CAD build for the part. Positions are in the model's coordinates, mm. A direction names the side the tool comes from. Round coordinates to 2 decimals unless told otherwise and drop trailing zeros. Write each loop counter-clockwise with the first axis right and the second up, starting at its lowest first coordinate (ties: lowest second). Pieces come first, ordered by that corner, then holes. Notation, with made-up numbers: (-37.75, 88) - (-26.75, 88) arc R6 cw to (-26.75, 92) - close; hole circle Ø3 at (43.25, 36). An arc over 180 degrees is marked (long way). Answer in a Markdown table with one row per item.
```python
from build123d import *

# Parameters (mm, degrees)
ESQUISSE1_W                  = 58.7375
ESQUISSE1_H                  = 15.24
BOSS_EXTRU_1_DEPTH           = 3.175
ESQUISSE1_3_W                = 4.7625
ESQUISSE1_3_H                = 15.24
BOSS_EXTRU_2_DEPTH           = 25.4
ENL_V_MAT_EXTRU_1_DEPTH      = 69.814783295
ENL_V_MAT_EXTRU_1_DEPTH_BACK = 69.814783295
CONG_1_R                     = 6.35
CONG_2_R                     = 1.27


with BuildPart() as part:
    # Esquisse1 → Boss.-Extru.1 (new body)
    with BuildSketch(Plane(origin=(0, 0, 0), x_dir=(1, 0, 0), z_dir=(0, 1, 0))):
        with Locations((2.38125, 0)):
            Rectangle(ESQUISSE1_W, ESQUISSE1_H)
        with BuildLine():
            ThreePointArc((19.05, 2.2479), (21.2979, 0), (19.05, -2.2479))
            Line((19.05, -2.2479), (-14.2875, -2.2479))
            ThreePointArc((-14.2875, -2.2479), (-16.5354, 0), (-14.2875, 2.2479))
            Line((-14.2875, 2.2479), (19.05, 2.2479))
        make_face(mode=Mode.SUBTRACT)
    extrude(amount=BOSS_EXTRU_1_DEPTH)

    # Esquisse1<3> → Boss.-Extru.2 (add)
    with BuildSketch(Plane(origin=(0, 0, 0), x_dir=(1, 0, 0), z_dir=(0, 1, 0))):
        with Locations((-29.36875, 0)):
            Rectangle(ESQUISSE1_3_W, ESQUISSE1_3_H)
    extrude(amount=BOSS_EXTRU_2_DEPTH)

    # Esquisse3 → Enlèv. mat.-Extru.1 (cut, two sides: drawn at the far end of the back side and taken through both)
    with BuildSketch(Plane.ZY.offset(31.75).offset(-ENL_V_MAT_EXTRU_1_DEPTH_BACK)):
        with BuildLine():
            Line((2.2479, 19.05), (2.2479, 9.525))
            ThreePointArc((2.2479, 9.525), (0, 7.2771), (-2.2479, 9.525))
            Line((-2.2479, 9.525), (-2.2479, 19.05))
            ThreePointArc((-2.2479, 19.05), (0, 21.2979), (2.2479, 19.05))
        make_face()
    extrude(amount=ENL_V_MAT_EXTRU_1_DEPTH + ENL_V_MAT_EXTRU_1_DEPTH_BACK, mode=Mode.SUBTRACT)

    # Congé1
    # the kernel refuses this fillet: 6.35 mm, written as the material it adds along each edge
    with BuildSketch(Plane(origin=(-26.9875, 3.175, -7.62), x_dir=(1, 0, 0), z_dir=(0, 0, 1))) as cong_1_piece_1_section:
        with BuildLine():
            CenterArc((CONG_1_R, CONG_1_R), CONG_1_R, 180, 90)
            Line((0, CONG_1_R), (0, 0))
            Line((0, 0), (CONG_1_R, 0))
        make_face()
    cong_1_piece_1 = extrude(amount=15.24, mode=Mode.PRIVATE)
    cong_1_piece_1 = cong_1_piece_1 - Plane(origin=(-25.549891024, 9.525, 0), x_dir=(0, 0, 1), z_dir=(1, 0, 0)) * Cylinder(2.2479, 56, mode=Mode.PRIVATE)
    add(cong_1_piece_1)
    # the kernel refuses this fillet: 6.35 mm, written as the material it takes off along each edge
    with BuildSketch(Plane(origin=(31.75, -15.875, 7.62), x_dir=(0, 0, -1), z_dir=(0, 1, 0)), Plane(origin=(31.75, -15.875, -7.62), x_dir=(-1, 0, 0), z_dir=(0, 1, 0))) as cong_1_2_piece_1:
        with BuildLine():
            CenterArc((CONG_1_R, CONG_1_R), CONG_1_R, 180, 90)
            Line((0, CONG_1_R), (0, 0))
            Line((0, 0), (CONG_1_R, 0))
        make_face()
    extrude(amount=34.925, mode=Mode.SUBTRACT)
    with BuildSketch(Plane(origin=(-11.1125, 25.4, -7.62), x_dir=(0, -1, 0), z_dir=(-1, 0, 0))) as cong_1_2_piece_2:
        with BuildLine():
            CenterArc((CONG_1_R, CONG_1_R), CONG_1_R, 180, 90)
            Line((0, CONG_1_R), (0, 0))
            Line((0, 0), (CONG_1_R, 0))
        make_face()
    extrude(amount=36.5125, mode=Mode.SUBTRACT)
    with BuildSketch(Plane(origin=(-47.625, 25.4, 7.62), x_dir=(0, 0, -1), z_dir=(1, 0, 0))) as cong_1_2_piece_3:
        with BuildLine():
            CenterArc((CONG_1_R, -CONG_1_R), CONG_1_R, 90, 90)
            Line((0, -CONG_1_R), (0, 0))
            Line((0, 0), (CONG_1_R, 0))
        make_face()
    extrude(amount=36.5125, mode=Mode.SUBTRACT)

    # Congé2
    cong_2_edges = [part.edges().sort_by_distance(p)[0] for p in [
        (-3.175, 0, -7.62),
        (-3.175, 0, 7.62),
        (-31.75, 0, 0),
        (2.38125, 3.175, 7.62),
        (31.75, 3.175, 0),
        (2.38125, 3.175, -7.62),
        (29.890128061, 3.175, -5.760128061),
        (29.890128061, 3.175, 5.760128061),
        (-26.9875, 14.2875, -7.62),
        (-26.9875, 25.4, 0),
        (-26.9875, 14.2875, 7.62),
        (-26.9875, 23.540128061, 5.760128061),
        (-26.9875, 23.540128061, -5.760128061),
        (31.75, 0, 0),
        (29.890128061, 0, -5.760128061),
        (29.890128061, 0, 5.760128061),
        (-31.75, 9.525, 7.62),
        (-31.75, 9.525, -7.62),
        (-31.75, 25.4, 0),
        (-31.75, 23.540128061, 5.760128061),
        (-31.75, 23.540128061, -5.760128061),
        (-25.127628061, 5.034871939, 7.62),
        (-25.127628061, 5.034871939, -7.62),
    ]]
    fillet(cong_2_edges, radius=CONG_2_R)


solid = part.part
```
Q1. Saw through at C-C on z = 0. Count the separate pieces of the cut face and the enclosed holes in it, then the cut area to 3 significant figures.
Computed:
| item | result |
|---|---|
| separate pieces | 3 |
| enclosed holes | 0 |
| area | 127 mm2 |
Q2. Drill centre lines: line 1 (X direction, y = 22.5, z = 1); line 2 (Z direction, x = 20.5, y = 3); line 3 (Y direction, x = 0, z = 4) (3 decimals). Where is each one in solid material? Low to high.
Computed:
| item | result |
|---|---|
| line 1 | x = -31.75 to -26.99 |
| line 2 | z = -6.99 to -1.72, 1.72 to 6.99 |
| line 3 | y = 0 to 3.175 |
Q3. Saw through at B-B on x = 3. List the corners of the cut face in (y, z) (3 decimals).
Computed:
| item | result |
|---|---|
| outline | (0, -6.35) arc R1.27 ccw to (1.27, -7.62) - (1.905, -7.62) arc R1.27 ccw to (3.175, -6.35) - (3.175, -2.248) - (0, -2.248) - close; (0, 2.248) - (3.175, 2.248) - (3.175, 6.35) arc R1.27 ccw to (1.905, 7.62) - (1.27, 7.62) arc R1.27 ccw to (0, 6.35) - close |
Q4. Pull direction Y, two halves, no side cores. Call faces 1 (the cylindrical face through (-29.4, 23.6, 5.7)), 2 (the flat face through (-26.987, 17, -3)), 3 (the cylindrical face through (-29.335, 21.297, -0.049)), 4 (the cylindrical face through (-29.127, 7.278, 0.049)): released by +Y, released by -Y, zero draft, split by the parting line, or undercut.
Computed:
| item | result |
|---|---|
| face 1 | released by +Y |
| face 2 | zero draft |
| face 3 | undercut |
| face 4 | undercut |
Q5. Flat gauge pins, fed straight in: pin 1 (4 mm diameter, centred on y = 17, z = 1, fed in from +X); pin 2 (6.5 mm diameter, centred on x = 14.5, z = -0.5, fed in from +Y) (3 decimals). Where does each tip first touch, or does it go through?
Computed:
| item | result |
|---|---|
| pin 1 | stops at x = -26.99 |
| pin 2 | stops at y = 3.175 |
Q6. Saw through at A-A on y = 15. List the corners of the cut face in (x, z).
Computed:
| item | result |
|---|---|
| outline | (-31.75, -6.35) arc R1.27 ccw to (-30.48, -7.62) - (-28.26, -7.62) arc R1.27 ccw to (-26.99, -6.35) - (-26.99, -2.25) - (-31.75, -2.25) - close; (-31.75, 2.25) - (-26.99, 2.25) - (-26.99, 6.35) arc R1.27 ccw to (-28.26, 7.62) - (-30.48, 7.62) arc R1.27 ccw to (-31.75, 6.35) - close |
Q7. 3-axis set-ups, long thin cutter, end or side, ignore diameter. For faces 5 (the flat face through (5, 3.175, -3)), 6 (the cylindrical face through (2.7, 2.81, 7.24)), 7 (the cylindrical face through (-31.368, 10.036, -7.258)): which of +Z, -Z, +X, -X, +Y, -Y reach the whole face in a straight line?
Computed:
| item | result |
|---|---|
| face 5 | +Z, -Z, +X, +Y |
| face 6 | +Z, +X, +Y |
| face 7 | -Z, -X, +Y, -Y |
